from build123d import *

# Parameters (mm, degrees)
SKETCH1_R           = 16
SKETCH1_R_2         = 2.25
BOSS_EXTRUDE1_DEPTH = 7.55
BOSS_EXTRUDE2_START = -7.55
BOSS_EXTRUDE2_DEPTH = 7.55
CIRPATTERN1_COUNT   = 10


with BuildPart() as part:
    # Sketch1 → Boss-Extrude1 (new body)
    with BuildSketch(Plane(origin=(0, 0, 0), x_dir=(1, 0, 0), z_dir=(0, 1, 0))):
        with Locations(Location((0, 0, 0), (0, 0, 270))):
            Circle(SKETCH1_R)
        with Locations(Location((0, 0, 0), (0, 0, 270))):
            Circle(SKETCH1_R_2, mode=Mode.SUBTRACT)
    extrude(amount=BOSS_EXTRUDE1_DEPTH)

    # Sketch2 → Boss-Extrude2 (add)
    with BuildSketch(Plane(origin=(0, 7.55, 0), x_dir=(1, 0, 0), z_dir=(0, 1, 0)).offset(BOSS_EXTRUDE2_START)):
        with BuildLine():
            Line((-1.403668826, 19.5), (1.403668826, 19.5))
            ThreePointArc((1.403668826, 19.5), (2.079259034, 19.237277337), (2.399863524, 18.587155743))
            Line((2.399863524, 18.587155743), (2.645477092, 15.779779813))
            ThreePointArc((2.645477092, 15.779779813), (0, 16), (-2.645477092, 15.779779813))
            Line((-2.645477092, 15.779779813), (-2.399863524, 18.587155743))
            ThreePointArc((-2.399863524, 18.587155743), (-2.079259034, 19.237277337), (-1.403668826, 19.5))
        make_face()
    boss_extrude2 = extrude(amount=BOSS_EXTRUDE2_DEPTH)

    # CirPattern1: Boss-Extrude2 ×10 about axis
    cirpattern1_axis = Axis((0, 0, 0), (0, 1, 0))
    for i in range(1, CIRPATTERN1_COUNT):
        add(boss_extrude2.rotate(cirpattern1_axis, i * 360 / CIRPATTERN1_COUNT))


solid = part.part
Could you check a few things on this model? Use its own coordinates, in mm. A direction names the side the tool comes from. Round coordinates to 2 decimals unless told otherwise and drop trailing zeros. Order: outer loops, then holes, each group sorted by start corner. A loop starts at its lowest first (then second) coordinate and runs counter-clockwise, first axis right, second up.
(1) Imagine slicing it at A-A (x = 0). Write out the boundary of the cut face in (y, z), plus the area to 3 significant figures.
Response values:
outline: (0, -19.5) - (7.55, -19.5) - (7.55, -2.25) - (0, -2.25) - close; (0, 2.25) - (7.55, 2.25) - (7.55, 19.5) - (0, 19.5) - close
area: 260 mm2
(2) If we mould it in two halves opening along Z, with no side actions, what happens to faces 1 (the flat face through (-18.55, 3.72, -6.01)), 2 (the cylindrical face through (9.636, 3.722, 16.787)), 3 (the flat face through (-12.13, 3.72, -12.4)), 4 (the flat face through (-4, 7.55, 0))? For each: released by +Z, released by -Z, zero draft, split by the parting line, or undercut.
Response values:
face 1: released by -Z
face 2: released by +Z
face 3: undercut
face 4: zero draft
(3) Imagine slicing it at C-C (x = -8). Write out the boundary of the cut face in (y, z).
Response values:
outline: (0, -15.32) - (7.55, -15.32) - (7.55, 15.32) - (0, 15.32) - close
(4) I'm going to push flat-ended pins straight in: pin 1 (2 mm diameter, centred on y = 1.5, z = -7, fed in from -X); pin 2 (1.5 mm diameter, centred on x = 5, z = -1.5, fed in from -Y); pin 3 (4 mm diameter, centred on y = 1, z = -10.5, fed in from +X); pin 4 (2 mm diameter, centred on x = 8, y = 3.5, fed in from +Z). Where does each tip first touch, or does it pass through?
Response values:
pin 1: stops at x = -18.55
pin 2: stops at y = 0
pin 3: stops at x = 13.56
pin 4: stops at z = 16.47
(5) Imagine slicing it at B-B (z = 0). Write out the boundary of the cut face in (x, y), plus the area to 3 significant figures.
Response values:
outline: (-16, 0) - (-2.25, 0) - (-2.25, 7.55) - (-16, 7.55) - close; (2.25, 0) - (16, 0) - (16, 7.55) - (2.25, 7.55) - close
area: 208 mm2
(6) Please list where these lines run through material, in increasing order: line 1 along X through (y, z) = (4.5, 16); line 2 along X through (y, z) = (1.25, -1); line 3 along X through (y, z) = (6.25, -2.5).
Response values:
line 1: x = -11.15 to -8.59, -2.63 to 2.63, 8.59 to 11.15
line 2: x = -15.97 to -2.02, 2.02 to 15.97
line 3: x = -16.15 to 16.15
(7) Imagine slicing it at D-D (x = 4). Write out the boundary of the cut face in (y, z), plus the area to 3 significant figures.
Response values:
outline: (0, -15.49) - (7.55, -15.49) - (7.55, 15.49) - (0, 15.49) - close
area: 234 mm2
(8) Which directions (+Z, -Z, +X, -X, +Y, -Y) give clear straight access to the entire face, cutting with the end or side of a thin tool? Please do faces 5 (the flat face through (-17.1, 3.7, -2.9)), 6 (the cylindrical face through (-5, 3.7, 15.2)), 7 (the cylindrical face through (18.943, 3.722, -3.977)).
Response values:
face 5: -X, +Y, -Y
face 6: +Z, +Y, -Y
face 7: +X, +Y, -Y
